Source: CAD feature listing. Evaluate the final solid. Frame: model axes, mm. A direction names the side the tool comes from. Round coordinates to 2 decimals unless told otherwise and drop trailing zeros. Order: outer loops, then holes, each group sorted by start corner. A loop starts at its lowest first (then second) coordinate and runs counter-clockwise, first axis right, second up. Notation, with made-up numbers: (-32, 89.5) -> (6, 89.5) arc R8 ccw to (6, 97.5) -> close; hole circle Ø10 at (-27.5, 85). An arc over 180 degrees is marked (long way). One line per item, written item: value. Start each with the question number.
1) Section A-A (z = 0). Return the cut outline in (x, y).
2) Section C-C (x = -56). Return the cut outline in (y, z), and give its area (3 significant figures).
3) Reachability of faces 1 (the face through (-84.21, 8.098, -18.436)), 2 (the face through (-131.075, 0.729, -9.032)), 3 (the face through (50.3, 6.1, 2)), 4 (the face through (41, 8, -30)), 5 (the face through (50.292, 9.352, 16.196)) from +Z, -Z, +X, -X, +Y, -Y: full face, straight path, thin tool, end or side. Return the list, or none.
4) Pin query (flat end, axial travel): P1, Ø4, axis at x = 46, y = 8, coming from the +Z side; P2, Ø17.5, axis at x = 46, y = 6.5, coming from the +Z side; P3, Ø24.5, axis at x = -61, z = 17.5, coming from the +Y side; P4, Ø8, axis at x = -143, z = 0, coming from the +Y side. Return the tip coordinate at first contact, or that it passes through.
5) Section B-B (x = 46). Return the cut outline in (y, z).
6) Ray query, L1, parallel to X at y = 3.5, z = 0; L2, parallel to Z at x = -143, y = 7; L3, parallel to Z at x = -139.5, y = 16. Return the intervals inside material, ascending.
7) Section D-D (x = -137). Return the cut outline in (y, z).
8) Mould query, pull axis Z, two halves, no side actions, for faces 6 (the face through (-34.4, 12, -14.4)), 7 (the face through (41, 8, 30)), 8 (the face through (42.86, 6.7, -16.2)), 9 (the face through (-85.42, 8.1, 18.22)). Classes: pulls with the +Z half, pulls with the -Z half, needs draft (parallel to the pull), parting line crosses it, or undercut.
```python
from build123d import *

# Parameters (mm, degrees)
EXTRUDE_1_DEPTH            = 16
CUT_EXTRUDE_1_DEPTH        = 140.143810498
CUT_EXTRUDE_1_DEPTH_BACK   = 140.143810498
SKETCH_2_R                 = 36
CUT_EXTRUDE_2_DEPTH        = 140.143810498
CUT_EXTRUDE_2_DEPTH_BACK   = 12
SKETCH_3_R                 = 38.5
CUT_EXTRUDE_1_2_DEPTH      = 140.143810498
CUT_EXTRUDE_1_2_DEPTH_BACK = 140.143810498
SKETCH_4_W                 = 46.223763545
SKETCH_4_H                 = 4
CUT_EXTRUDE_3_REACH        = 152.735
SKETCH_5_R                 = 4.5
HOLE_WIZARD_M8_1_D         = 6.8
FILLET_1_R                 = 10
EXTRUDE_2_DEPTH            = 22
CUT_EXTRUDE_4_REACH        = 162.378
CHAMFER_1_SIZE             = 1
CHAMFER_2_SIZE             = 1
CUT_EXTRUDE_5_REACH        = 218.649
SKETCH_12_R                = 7.5
F_5_0MM_1_D                = 5
CHAMFER_3_SIZE             = 1


with BuildPart() as part:
    # 草图1 → 凸台-拉伸1 (new body)
    with BuildSketch(Plane(origin=(0, 0, 0), x_dir=(1, 0, 0), z_dir=(0, 1, 0))):
        with BuildLine():
            Line((56, 30), (27.946377225, 30))
            ThreePointArc((27.946377225, 30), (11.579874692, 39.330732286), (-7.231593148, 40.357205807))
            Line((-7.231593148, 40.357205807), (-132, 18))
            Line((-132, 18), (-132, -18))
            Line((-132, -18), (-7.231593148, -40.357205807))
            ThreePointArc((-7.231593148, -40.357205807), (11.579874692, -39.330732286), (27.946377225, -30))
            Line((27.946377225, -30), (56, -30))
            Line((56, -30), (56, 30))
        make_face()
    extrude(amount=EXTRUDE_1_DEPTH)

    # 草图2 → Cut-Extrude 1 (cut, two sides: drawn at the far end of the back side and taken through both)
    with BuildSketch(Plane(origin=(0, 16, 0), x_dir=(1, 0, 0), z_dir=(0, 1, 0)).offset(-CUT_EXTRUDE_1_DEPTH_BACK)):
        with Locations(Location((0, 0, 0), (0, 0, 270))):
            Circle(SKETCH_2_R)
    extrude(amount=CUT_EXTRUDE_1_DEPTH + CUT_EXTRUDE_1_DEPTH_BACK, mode=Mode.SUBTRACT)

    # 草图3 → 切除-拉伸2 (cut, two sides: drawn at the far end of the back side and taken through both)
    with BuildSketch(Plane.XZ.offset(-CUT_EXTRUDE_2_DEPTH_BACK)):
        with Locations(Location((0, 0, 0), (0, 0, 90))):
            Circle(SKETCH_3_R)
    extrude(amount=CUT_EXTRUDE_2_DEPTH + CUT_EXTRUDE_2_DEPTH_BACK, mode=Mode.SUBTRACT)

    # 草图4 → Cut-Extrude 1 2 (cut, two sides: drawn at the far end of the back side and taken through both)
    with BuildSketch(Plane(origin=(0, 16, 0), x_dir=(1, 0, 0), z_dir=(0, 1, 0)).offset(-CUT_EXTRUDE_1_2_DEPTH_BACK)):
        with Locations((51.058258998, 0)):
            Rectangle(SKETCH_4_W, SKETCH_4_H)
    extrude(amount=CUT_EXTRUDE_1_2_DEPTH + CUT_EXTRUDE_1_2_DEPTH_BACK, mode=Mode.SUBTRACT)

    # 草图5 → 切除-拉伸3 (cut, up to next)
    with BuildSketch(Plane.XY.offset(30), mode=Mode.PRIVATE) as cut_extrude_3_sk1:
        with Locations((46, 8)):
            Circle(SKETCH_5_R)
    cut_extrude_3_tool1 = extrude(cut_extrude_3_sk1.sketch, amount=-CUT_EXTRUDE_3_REACH, mode=Mode.PRIVATE) & part.part
    add(cut_extrude_3_tool1.solids().sort_by_distance((46, 8, 30))[0], mode=Mode.SUBTRACT)

    # M8 螺纹孔1 (through all)
    with Locations(Plane.XY.offset(-2)):
        with Locations((46, 8)):
            Hole(HOLE_WIZARD_M8_1_D / 2)

    # 圆角1
    fillet_1_edges = [part.edges().sort_by_distance(p)[0] for p in [
        (27.946377225, 8, 30),
        (27.946377225, 8, -30),
    ]]
    fillet(fillet_1_edges, radius=FILLET_1_R)

    # 草图11 → 凸台-拉伸2 (add)
    with BuildSketch(Plane.ZY.offset(132)):
        with BuildLine():
            Line((-18, 0), (18, 0))
            Line((18, 0), (18, 16))
            ThreePointArc((18, 16), (0, 34), (-18, 16))
            Line((-18, 16), (-18, 0))
        make_face()
    extrude(amount=EXTRUDE_2_DEPTH)

    # 草图13 → 切除-拉伸4 (cut, up to next)
    with BuildSketch(Plane(origin=(0, 16, 0), x_dir=(1, 0, 0), z_dir=(0, 1, 0)), mode=Mode.PRIVATE) as cut_extrude_4_sk1:
        with BuildLine():
            Line((-41.744935847, 26.04535143), (-127.881901603, 10.610499615))
            ThreePointArc((-127.881901603, 10.610499615), (-130.834677823, 8.897509725), (-132, 5.688889151))
            Line((-132, 5.688889151), (-132, -5.688889151))
            ThreePointArc((-132, -5.688889151), (-130.834677823, -8.897509725), (-127.881901603, -10.610499615))
            Line((-127.881901603, -10.610499615), (-41.744935847, -26.04535143))
            ThreePointArc((-41.744935847, -26.04535143), (-36.839154105, -24.091633928), (-36.421400087, -18.827682165))
            ThreePointArc((-36.421400087, -18.827682165), (-41, 0), (-36.421400087, 18.827682165))
            ThreePointArc((-36.421400087, 18.827682165), (-36.839154105, 24.091633928), (-41.744935847, 26.04535143))
        make_face()
    cut_extrude_4_tool1 = extrude(cut_extrude_4_sk1.sketch, amount=-CUT_EXTRUDE_4_REACH, mode=Mode.PRIVATE) & part.part
    add(cut_extrude_4_tool1.solids().sort_by_distance((-78.107907, 16, 0))[0], mode=Mode.SUBTRACT)

    # 倒角1
    chamfer_1_edges = [part.edges().sort_by_distance(p)[0] for p in [
        (-130.834677823, 16, -8.897509725),
        (-130.834677823, 16, 8.897509725),
        (-84.813418725, 16, 18.327925523),
        (-36.839154105, 16, 24.091633928),
        (-41, 16, 0),
        (-36.839154105, 16, -24.091633928),
        (-84.813418725, 16, -18.327925523),
        (-132, 0, 0),
        (-130.834677823, 0, -8.897509725),
        (-84.813418725, 0, -18.327925523),
        (-36.839154105, 0, -24.091633928),
        (-41, 0, 0),
        (-36.839154105, 0, 24.091633928),
        (-84.813418725, 0, 18.327925523),
        (-130.834677823, 0, 8.897509725),
    ]]
    chamfer(chamfer_1_edges, length=CHAMFER_1_SIZE)

    # 倒角2
    chamfer_2_edges = [part.edges().sort_by_distance(p)[0] for p in [
        (-26.153393661, 12, -24.738633754),
    ]]
    chamfer(chamfer_2_edges, length=CHAMFER_2_SIZE)

    # 草图12 → 切除-拉伸5 (cut, up to next)
    with BuildSketch(Plane.ZY.offset(154), mode=Mode.PRIVATE) as cut_extrude_5_sk1:
        with Locations((0, 16)):
            Circle(SKETCH_12_R)
    cut_extrude_5_tool1 = extrude(cut_extrude_5_sk1.sketch, amount=-CUT_EXTRUDE_5_REACH, mode=Mode.PRIVATE) & part.part
    add(cut_extrude_5_tool1.solids().sort_by_distance((-154, 16, 0))[0], mode=Mode.SUBTRACT)

    # Ø5.0mm 暗销孔1 (through all)
    with Locations(Plane(origin=(-143, 34, 0), x_dir=(0, 0, 1), z_dir=(0, 1, 0))):
        with Locations((0, 0)):
            Hole(F_5_0MM_1_D / 2)

    # 倒角3
    chamfer_3_edges = [part.edges().sort_by_distance(p)[0] for p in [
        (-154, 16, -7.5),
    ]]
    chamfer(chamfer_3_edges, length=CHAMFER_3_SIZE)


solid = part.part
```
Findings:
1. outline: (-154, 0) -> (-145.5, 0) -> (-145.5, 8.5) -> (-153, 8.5) -> (-154, 7.5) -> close; (-154, 24.5) -> (-153, 23.5) -> (-145.5, 23.5) -> (-145.5, 34) -> (-154, 34) -> close; (-140.5, 0) -> (-133, 0) -> (-132, 1) -> (-132, 8.5) -> (-140.5, 8.5) -> close; (-140.5, 23.5) -> (-132, 23.5) -> (-132, 34) -> (-140.5, 34) -> close; (-41, 1) -> (-40, 0) -> (-38.5, 0) -> (-38.5, 12) -> (-37, 12) -> (-36, 13) -> (-36, 16) -> (-40, 16) -> (-41, 15) -> close
2. outline: (0, -31.62) -> (16, -31.62) -> (16, -24.51) -> (15, -23.49) -> (1, -23.49) -> (0, -24.51) -> close; (0, 24.51) -> (1, 23.49) -> (15, 23.49) -> (16, 24.51) -> (16, 31.62) -> (0, 31.62) -> close
2. area: 258 mm2
3. face 1: +Y, -Y
3. face 2: -Y
3. face 3: +X, +Y, -Y
3. face 4: -Z, +X, +Y, -Y
3. face 5: +Z
4. P1: through
4. P2: z = 30
4. P3: y = 16
4. P4: y = 34
5. outline: (0, -30) -> (4.6, -30) -> (4.6, -2) -> (0, -2) -> close; (0, 2) -> (3.5, 2) -> (3.5, 30) -> (0, 30) -> close; (11.4, -30) -> (16, -30) -> (16, -2) -> (11.4, -2) -> close; (12.5, 2) -> (16, 2) -> (16, 30) -> (12.5, 30) -> close
6. L1: -154 to -145.5, -140.5 to -132, -41 to -38.5
6. L2: -18 to -2.5, 2.5 to 18
6. L3: -18 to -7.5, 7.5 to 18
7. outline: (0, -18) -> (16, -18) arc R18 ccw to (16, 18) -> (0, 18) -> close; hole circle Ø15 at (16, 0)
8. face 6: undercut
8. face 7: pulls with the +Z half
8. face 8: needs draft
8. face 9: undercut
